Source: CAD feature listing. Evaluate the final solid. Frame: model axes, mm. A direction names the side the tool comes from. Give positions to 0.01 mm unless a question says otherwise; leave off trailing zeros. Order: outer loops, then holes, each group sorted by start corner. A loop starts at its lowest first (then second) coordinate and runs counter-clockwise, first axis right, second up. Notation, with made-up numbers: (31, 37.5) -> (42, 37.5) arc R27 cw to (42, 53.5) -> close; hole circle Ø9 at (3.5, 43). An arc over 180 degrees is marked (long way). Answer in a Markdown table with one row per item.
```python
from build123d import *

# Parameters (mm, degrees)
SKETCH1_R           = 15
SKETCH1_R_2         = 6.25
BOSS_EXTRUDE1_DEPTH = 10
SKETCH2_R           = 15
SKETCH2_R_2         = 12.5
BOSS_EXTRUDE2_DEPTH = 20
CUT_EXTRUDE1_DEPTH  = 37.742346142
BOSS_EXTRUDE3_DEPTH = 25
SKETCH5_R           = 1.5
CUT_EXTRUDE2_DEPTH  = 48.563115962
CUT_EXTRUDE3_DEPTH  = 35.441980199
CHAMFER2_SIZE       = 2


with BuildPart() as part:
    # Sketch1 → Boss-Extrude1 (new body)
    with BuildSketch(Plane(origin=(0, 0, 0), x_dir=(1, 0, 0), z_dir=(0, 1, 0))):
        with Locations(Location((0, 0, 0), (0, 0, 270))):
            Circle(SKETCH1_R)
        with Locations(Location((0, 0, 0), (0, 0, 270))):
            Circle(SKETCH1_R_2, mode=Mode.SUBTRACT)
    extrude(amount=BOSS_EXTRUDE1_DEPTH)

    # Sketch2 → Boss-Extrude2 (add)
    with BuildSketch(Plane(origin=(0, 10, 0), x_dir=(1, 0, 0), z_dir=(0, 1, 0))):
        with Locations(Location((0, 0, 0), (0, 0, 270))):
            Circle(SKETCH2_R)
        with Locations(Location((0, 0, 0), (0, 0, 270))):
            Circle(SKETCH2_R_2, mode=Mode.SUBTRACT)
    extrude(amount=BOSS_EXTRUDE2_DEPTH)

    # Sketch3 → Cut-Extrude1 (cut, through all)
    with BuildSketch(Plane(origin=(0, 0, 0), x_dir=(1, 0, 0), z_dir=(0, 1, 0))):
        with BuildLine():
            Line((0, 0), (-9.641814145, 11.490666647))
            ThreePointArc((-9.641814145, 11.490666647), (-15, 0), (-9.641814145, -11.490666647))
            Line((-9.641814145, -11.490666647), (0, 0))
        make_face()
    extrude(amount=CUT_EXTRUDE1_DEPTH, mode=Mode.SUBTRACT)

    # Sketch4 → Boss-Extrude3 (add)
    with BuildSketch(Plane(origin=(0, 0, 0), x_dir=(1, 0, 0), z_dir=(0, 1, 0))):
        with BuildLine():
            Line((-9.641814145, 11.490666647), (-9.641814145, 15))
            Line((-9.641814145, 15), (-21.5, 15))
            Line((-21.5, 15), (-21.5, 18))
            Line((-21.5, 18), (3.5, 18))
            Line((3.5, 18), (10.811384743, 10.3977863))
            ThreePointArc((10.811384743, 10.3977863), (0.800356614, 14.978632424), (-9.641814145, 11.490666647))
        make_face()
    extrude(amount=BOSS_EXTRUDE3_DEPTH)

    # Sketch5 → Cut-Extrude2 (cut, through all)
    with BuildSketch(Plane.XY.offset(-15)):
        with Locations((-17.5, 20)):
            Circle(SKETCH5_R)
        with Locations((-17.5, 10)):
            Circle(SKETCH5_R)
    extrude(amount=-CUT_EXTRUDE2_DEPTH, mode=Mode.SUBTRACT)

    # Sketch6 → Cut-Extrude3 (cut, through all)
    with BuildSketch(Plane(origin=(0, 10, 0), x_dir=(1, 0, 0), z_dir=(0, 1, 0))):
        with BuildLine():
            Line((0, -6.25), (-12.5, -6.25))
            ThreePointArc((-12.5, -6.25), (-18.75, 0), (-12.5, 6.25))
            Line((-12.5, 6.25), (0, 6.25))
            ThreePointArc((0, 6.25), (6.25, 0), (0, -6.25))
        make_face()
    extrude(amount=-CUT_EXTRUDE3_DEPTH, mode=Mode.SUBTRACT)

    # Chamfer2
    chamfer2_edges = [part.edges().sort_by_distance(p)[0] for p in [
        (-8.838329633, 30, -10.533111093),
        (-8.838329633, 30, 10.533111093),
        (-21.5, 25, -16.5),
    ]]
    chamfer(chamfer2_edges, length=CHAMFER2_SIZE)


solid = part.part
```
(1) Section query A-A (y = 20). Return the cut outline in (x, z).
A:
| item | result |
|---|---|
| outline | (-21.5, -18) -> (-19, -18) -> (-19, -15) -> (-21.5, -15) -> close; (-16, -18) -> (3.5, -18) -> (10.81, -10.4) arc R15 ccw to (-9.64, 11.49) -> (-8.03, 9.58) arc R12.5 cw (long way) to (-8.03, -9.58) -> (-9.64, -11.49) -> (-9.64, -15) -> (-16, -15) -> close |
(2) Section query C-C (x = 2). Return the cut outline in (y, z), plus the area to 3 significant figures.
A:
| item | result |
|---|---|
| outline | (0, -18) -> (25, -18) -> (25, -14.87) -> (30, -14.87) -> (30, -12.34) -> (10, -12.34) -> (10, -5.92) -> (0, -5.92) -> close; (0, 5.92) -> (10, 5.92) -> (10, 12.34) -> (30, 12.34) -> (30, 14.87) -> (0, 14.87) -> close |
| area | 358 mm^2 |
(3) Ray query, probe 1 along Y at (x, z) = (-17.5, -16.65); probe 2 along Z at (x, y) = (0, 18); probe 3 along Y at (x, z) = (-4, -8). Return the intervals inside material, ascending.
A:
| item | result |
|---|---|
| probe 1 | y = 0 to 8.5, 11.5 to 18.5, 21.5 to 25 |
| probe 2 | z = -18 to -12.5, 12.5 to 15 |
| probe 3 | y = 0 to 10 |
(4) First-contact query: pin 1 Ø6 at (x, z) = (5, -2.5) entering from +Y; pin 2 Ø2.5 at (x, y) = (-2, 7) entering from +Z; pin 3 Ø1.1 at (y, z) = (14.5, -14) entering from -X. Flat tips, straight axial feed; report the tip coordinate or a pass-through.
A:
| item | result |
|---|---|
| pin 1 | stops at y = 10 |
| pin 2 | stops at z = 14.98 |
| pin 3 | stops at x = -9.64 |
(5) Section query D-D (y = 12.25). Return the cut outline in (x, z).
A:
| item | result |
|---|---|
| outline | (-21.5, -18) -> (3.5, -18) -> (10.81, -10.4) arc R15 ccw to (-9.64, 11.49) -> (-8.03, 9.58) arc R12.5 cw (long way) to (-8.03, -9.58) -> (-9.64, -11.49) -> (-9.64, -15) -> (-21.5, -15) -> close |
(6) Pull-direction query (X, two-part tool) for faces 1 (the flat face through (-8.022, 29.014, -11.137)), 2 (the cylindrical face through (-19, 10, -16)), 3 (the cylindrical face through (12.897, 14.79, 7.66)), 4 (the flat face through (-15, 12, -15)); classes: +X half, -X half, draft (parallel to the pull), parting line (faces both ways), or undercut.
A:
| item | result |
|---|---|
| face 1 | -X half |
| face 2 | undercut |
| face 3 | parting line |
| face 4 | draft |
(7) Access query for faces 5 (the flat face through (-8.019, 28.986, 11.091)), 6 (the flat face through (7, 10, 0)), 7 (the flat face through (-9.642, 12, -13)), 8 (the flat face through (-8.45, 10.69, 10.07)). Directions: +Z, -Z, +X, -X, +Y, -Y. A direction counts if a zero-diameter tool reaches every point of the face in a straight line with its end or side. Return the directions, or none.
A:
| item | result |
|---|---|
| face 5 | -X, +Y |
| face 6 | +Y |
| face 7 | +Z, -X, +Y, -Y |
| face 8 | -X, +Y, -Y |
(8) Section query B-B (x = -17.5). Return the cut outline in (y, z), plus the area to 3 significant figures.
A:
| item | result |
|---|---|
| outline | (0, -18) -> (8.5, -18) -> (8.5, -15) -> (0, -15) -> close; (11.5, -18) -> (18.5, -18) -> (18.5, -15) -> (11.5, -15) -> close; (21.5, -18) -> (25, -18) -> (25, -15) -> (21.5, -15) -> close |
| area | 57.0 mm^2 |
